The listing builds one solid part. Answer for the finished solid, in the listing's coordinates (mm). A direction names the side the tool comes from. Coordinates: 2 decimals unless noted, no trailing zeros. Loops run counter-clockwise (first coordinate to the right, second up) from the corner with the lowest first, then second, coordinate; pieces in that order, holes last. Notation, with made-up numbers: (-36.75, 43) - (15.25, 43) arc R9 ccw to (15.25, 58) - close; hole circle Ø8 at (82, -15.75). An arc over 180 degrees is marked (long way). Return JSON: item names as keys, results as strings. Group by question number.
1. Find the intervals of material crossed by line 1 along Z through (x, y) = (1, -9.25); line 2 along X through (y, z) = (-8.75, 30); line 3 along Y through (x, z) = (64, 23.5), in increasing order.
2. Each of these flat-tipped pins is pushed along its axis until it touches: P1, Ø3, axis at y = -10, z = -3, coming from the +X side; P2, Ø2.5, axis at x = -39.5, z = 23, coming from the -Y side; P3, Ø3.5, axis at x = -102, z = -5, coming from the -Y side; P4, Ø3, axis at y = -9.5, z = 5, coming from the -X side. Where does it stop, or does it pass through?
3. Section A-A (z = 13) is taken. Write down the section's boundary in (x, y).
4. Which of the six approach directions +Z, -Z, +X, -X, +Y, -Y give full straight-line access (tool end or side, diameter ignored) to faces 1 (the face through (-104, -6, 0)), 2 (the face through (-2, 0, 0)), 3 (the face through (104, -6, 0))?
```python
from build123d import *

# Parameters (mm, degrees)
F0_W     = 220
F0_H     = 68
F1_DEPTH = 12
F2_W     = 3
F2_H     = 3
F3_DEPTH = 300
F4_W     = 12
F4_H     = 68
F5_DEPTH = 6


with BuildPart() as f1:
    # F0 (on Front) → F1 (new body)
    with BuildSketch(Plane.XZ):
        Rectangle(F0_W, F0_H)
    extrude(amount=F1_DEPTH)

    # F2 (on face) → F3 (cut)
    with BuildSketch(Plane(origin=(-110, 0, 0), x_dir=(0, -1, 0), z_dir=(-1, 0, 0))):
        with Locations((10.5, 22.5)):
            Rectangle(F2_W, F2_H)
    extrude(amount=-F3_DEPTH, mode=Mode.SUBTRACT)

    # F4 (on face) → F5 (cut)
    with BuildSketch(Plane.XZ.offset(12)):
        with Locations((-104.358618, 0)):
            Rectangle(F4_W, F4_H)
        with Locations((104, 0)):
            Rectangle(F4_W, F4_H)
    extrude(amount=-F5_DEPTH, mode=Mode.SUBTRACT)


solid = f1.part
```
The answers:
{
 "1": {"line 1": "z = -34 to 21, 24 to 34", "line 2": "x = -98.36 to 98", "line 3": "y = -9 to 0"},
 "2": {"P1": "stops at x = 98", "P2": "stops at y = -12", "P3": "stops at y = -6", "P4": "stops at x = -98.36"},
 "3": {"outline": "(-110, -6) - (-98.36, -6) - (-98.36, -12) - (98, -12) - (98, -6) - (110, -6) - (110, 0) - (-110, 0) - close"},
 "4": {"face 1": "+Z, -Z, -X, -Y", "face 2": "+Z, -Z, +X, -X, +Y", "face 3": "+Z, -Z, +X, -Y"}
}
